```python
from build123d import *

# Parameters (mm, degrees)
SKIZZE1_W                       = 47.8
SKIZZE1_H                       = 9.6
AUFSATZ_LINEAR_AUSTRAGEN1_DEPTH = 4
SKIZZE2_R                       = 2.45
SCHNITT_LINEAR_AUSTRAGEN1_DEPTH = 9
SKIZZE2_3_R                     = 3
SKIZZE2_3_R_2                   = 2.45
SCHNITT_LINEAR_AUSTRAGEN2_DEPTH = 0.9
M2_GEWINDEBOHRUNG1_D            = 1.6
SKIZZE5_R                       = 2.45
SCHNITT_LINEAR_AUSTRAGEN3_DEPTH = 2


with BuildPart() as part:
    # Skizze1 → Aufsatz-Linear austragen1 (new body, symmetric)
    with BuildSketch(Plane.XY):
        Rectangle(SKIZZE1_W, SKIZZE1_H)
    extrude(amount=AUFSATZ_LINEAR_AUSTRAGEN1_DEPTH, both=True)

    # Skizze2 → Schnitt-Linear austragen1 (cut, through all)
    with BuildSketch(Plane.XY.offset(4)):
        with Locations((-16, 0.95)):
            Circle(SKIZZE2_R)
        with Locations((0, 0.95)):
            Circle(SKIZZE2_R)
        with Locations((16, 0.95)):
            Circle(SKIZZE2_R)
    extrude(amount=-SCHNITT_LINEAR_AUSTRAGEN1_DEPTH, mode=Mode.SUBTRACT)

    # Skizze2_3 → Schnitt-Linear austragen2 (cut)
    with BuildSketch(Plane.XY.offset(4)):
        with Locations((-16, 0.95)):
            Circle(SKIZZE2_3_R)
        with Locations((-16, 0.95)):
            Circle(SKIZZE2_3_R_2, mode=Mode.SUBTRACT)
        with Locations((0, 0.95)):
            Circle(SKIZZE2_3_R)
        with Locations((0, 0.95)):
            Circle(SKIZZE2_3_R_2, mode=Mode.SUBTRACT)
        with Locations((16, 0.95)):
            Circle(SKIZZE2_3_R)
        with Locations((16, 0.95)):
            Circle(SKIZZE2_3_R_2, mode=Mode.SUBTRACT)
    schnitt_linear_austragen2 = extrude(amount=-SCHNITT_LINEAR_AUSTRAGEN2_DEPTH, mode=Mode.SUBTRACT)

    # Spiegeln1: Schnitt-Linear austragen2 across plane
    add(schnitt_linear_austragen2.mirror(Plane.XY), mode=Mode.SUBTRACT)

    # M2 Gewindebohrung1 (through all)
    with Locations(Plane(origin=(0, -4.8, 0), x_dir=(-1, 0, 0), z_dir=(0, -1, 0))):
        with Locations((-8, 0), (8, 0)):
            Hole(M2_GEWINDEBOHRUNG1_D / 2)

    # Skizze5 → Schnitt-Linear austragen3 (cut)
    with BuildSketch(Plane.XZ.offset(4.8)):
        with Locations((-20, 0)):
            Circle(SKIZZE5_R)
        with Locations((-4, 0)):
            Circle(SKIZZE5_R)
        with Locations((-12, 0)):
            Circle(SKIZZE5_R)
        with Locations((4, 0)):
            Circle(SKIZZE5_R)
        with Locations((12, 0)):
            Circle(SKIZZE5_R)
        with Locations((20, 0)):
            Circle(SKIZZE5_R)
    extrude(amount=-SCHNITT_LINEAR_AUSTRAGEN3_DEPTH, mode=Mode.SUBTRACT)


solid = part.part
```
Work out the finished part from the listing and answer in its coordinate system (mm). A direction names the side the tool comes from. Coordinates: 2 decimals unless noted, no trailing zeros. Order: outer loops, then holes, each group sorted by start corner. A loop starts at its lowest first (then second) coordinate and runs counter-clockwise, first axis right, second up. Notation, with made-up numbers: (16.25, -14) - (59.25, -14) arc R21 ccw to (59.25, -4) - close; hole circle Ø2 at (19, 3). An arc over 180 degrees is marked (long way). Answer as a JSON object with one key per item and string values.
1. The mould has two halves that part along Y. Classify faces 4 (the face through (-18.997, 1.082, -3.556)), 5 (the face through (13.003, 1.082, 3.556)), 6 (the face through (17.552, -3.814, 0.108)), 7 (the face through (-12, -2.8, 0)): +Y half, -Y half, draft (parallel to the pull), parting line (faces both ways), or undercut.
Output values:
{"face 4": "undercut", "face 5": "undercut", "face 6": "draft", "face 7": "-Y half"}
2. Each of these flat-tipped pins is pushed along its axis until it touches: P1, Ø3, axis at x = 1, y = 0.5, coming from the -Z side; P2, Ø1.5, axis at x = -4, z = 2, coming from the -Y side; P3, Ø3, axis at x = -12, z = 0, coming from the -Y side. Where does it stop, or does it pass through?
Output values:
{"P1": "stops at z = -3.1", "P2": "stops at y = -4.8", "P3": "stops at y = -2.8"}
3. A tool of negligible diameter and unlimited length cuts with its end or side. For faces 1 (the face through (-1.663, -3.814, 0.736)), 2 (the face through (-2.997, 1.082, 3.556)), 3 (the face through (-8.8, 0.1, 0)), from which of +Z, -Z, +X, -X, +Y, -Y can it reach the whole face along a straight path? Write none if from no direction.
Output values:
{"face 1": "-Y", "face 2": "+Z", "face 3": "+Y, -Y"}
4. Find section A-A on x = 0. Determine the outline of the cut face in (y, z).
Output values:
{"outline": "(-4.8, -4) - (-2.05, -4) - (-2.05, -3.1) - (-1.5, -3.1) - (-1.5, 3.1) - (-2.05, 3.1) - (-2.05, 4) - (-4.8, 4) - close; (3.4, -3.1) - (3.95, -3.1) - (3.95, -4) - (4.8, -4) - (4.8, 4) - (3.95, 4) - (3.95, 3.1) - (3.4, 3.1) - close"}
5. Find section B-B on y = -3.25. Count the separate pieces of the cut face and the enclosed holes in it, plus the area to 3 significant figures.
Output values:
{"separate pieces": "1", "enclosed holes": "8", "area": "265 mm²"}
6. Find section D-D on x = 12. Determine the outline of the cut face in (y, z), plus the area to 3 significant figures.
Output values:
{"outline": "(-4.8, -4) - (4.8, -4) - (4.8, 4) - (-4.8, 4) - (-4.8, 2.45) - (-2.8, 2.45) - (-2.8, -2.45) - (-4.8, -2.45) - close", "area": "67.0 mm²"}
7. Consider line 1 (X direction, y = 1.5, z = 3); line 2 (Z direction, x = -20, y = -4.2); line 3 (Z direction, x = 8, y = 0.5). Determine where each line is inside the solid, lowest interval first.
Output values:
{"line 1": "x = -23.9 to -18.39, -13.61 to -2.39, 2.39 to 13.61, 18.39 to 23.9", "line 2": "z = -4 to -2.45, 2.45 to 4", "line 3": "z = -4 to -0.8, 0.8 to 4"}
